Verification items for the finished model (mm, model axes). A direction names the side the tool comes from. Give positions to 0.01 mm unless a question says otherwise; leave off trailing zeros. Loops run counter-clockwise (first coordinate to the right, second up) from the corner with the lowest first, then second, coordinate; pieces in that order, holes last. Notation, with made-up numbers: (56, 37) - (63, 37) arc R21 ccw to (63, 41) - close; hole circle Ø11 at (-12, 60). An arc over 180 degrees is marked (long way). One line per item, written item: value. Start each with the question number.
1. Access from +Z, -Z, +X, -X, +Y, -Y to the whole of each face (thin tool, end or side, straight path). Record for faces 1 (the cylindrical face through (4.36, 2.45, 3.61)), 2 (the cylindrical face through (-0.1, -5, 3.6)), 3 (the flat face through (-0.1, -5.2, 3.2)), 4 (the cylindrical face through (-0.534, 4.065, 0.109)).
2. Scan lines: L1, parallel to Y at x = 0, z = 0.3; L2, parallel to Z at x = 2.5, y = -2; L3, parallel to X at y = -2.25, z = 0.35. Record each from-to range of solid material in increasing order. Write a range as [from, to].
3. Gauge pin test, flat ends, axial feed: pin 1 (1 mm diameter, centred on x = 1, z = 0, fed in from -Y); pin 2 (2 mm diameter, centred on y = 2, z = 0, fed in from -X); pin 3 (4.5 mm diameter, centred on x = 0, y = 6, fed in from -Z); pin 4 (2 mm diameter, centred on x = 0, y = 0, fed in from +Z). Record the tip position at first contact, or that the pin passes through.
4. Sectioned sample at A-A (x = 0). Count the separate pieces of the cut face and the enclosed holes in it, plus the area to 3 significant figures.
5. Mould release check, pull along X, two halves, no side actions. Record for faces 5 (the cylindrical face through (-4.3, 2.55, 3.61)), 6 (the flat face through (1, -1, 4)), 7 (the flat face through (-1, -1, 1.25)): pulls with the +X half, pulls with the -X half, needs draft (parallel to the pull), parting line crosses it, or undercut.
6. Sectioned sample at C-C (z = 2). Record the cut outline in (x, y).
from build123d import *

# Parameters (mm, degrees)
CYLINDER001_R     = 1.35
CYLINDER001_DEPTH = 10
ARRAY001_COUNT    = 3
CYLINDER_R        = 4.1
CYLINDER_DEPTH    = 2.25
SKETCH002_W       = 5
SKETCH002_H       = 4.7
ARRAY_Z_COUNT     = 6
ARRAY_Z_PITCH     = 1.6


with BuildPart() as obj1:
    # Cylinder001 → Cylinder001 (new body)
    with BuildSketch(Plane(origin=(0, 6, -4), x_dir=(1, 0, 0), z_dir=(0, 0, 1))):
        Circle(CYLINDER001_R)
    extrude(amount=CYLINDER001_DEPTH)

    # Array001: obj1 ×3 about axis
    array001_axis = Axis((0, 0, 0), (0, 0, 1))


with BuildPart() as obj1_1:
    add(obj1.part)
    for i in range(1, ARRAY001_COUNT):
        add(obj1.part.rotate(array001_axis, i * 360 / ARRAY001_COUNT))


with BuildPart() as lensfit:
    # Cylinder → Cylinder (new body)
    with BuildSketch(Plane.XY.offset(-1)):
        Circle(CYLINDER_R)
    extrude(amount=CYLINDER_DEPTH)


with BuildPart() as obj2:
    # Sketch002 → Revolution002 (revolve)
    with BuildSketch(Plane.XZ):
        with Locations((7.5, 0.85)):
            Rectangle(SKETCH002_W, SKETCH002_H)
    revolve(axis=Axis((0, 0, 0), (0, 0, 1)))


with BuildPart() as innergroovetool:
    # Sketch001 → Revolution001 (revolve)
    with BuildSketch(Plane.XZ):
        Polygon((4, 3.2), (4, 1.6), (8, 1.6), (8.8, 2.4), (8, 3.2), align=None)
    revolve(axis=Axis((0, 0, 0), (0, 0, 1)))

    # Array Z: InnerGrooveTool ×6


with BuildPart() as innergroovetool_1:
    add(innergroovetool.part)
    with Locations(*[(0, 0, -i * ARRAY_Z_PITCH) for i in range(1, ARRAY_Z_COUNT)]):
        add(innergroovetool.part)

    # Common: intersect obj2
    add(obj2.part, mode=Mode.INTERSECT)


with BuildPart() as boltcuts:
    # Sketch → Revolution (revolve)
    with BuildSketch(Plane.XZ):
        Polygon((1.25, 4), (1.25, -1.5), (8, -1.5), (8, 3.2), (5, 3.2), (5, 4), align=None)
    revolve(axis=Axis((0, 0, 0), (0, 0, 1)))

    # Fusion001: union InnerGrooveTool
    add(innergroovetool_1.part)

    # Cut: cut LensFit
    add(lensfit.part, mode=Mode.SUBTRACT)

    # Cut001: cut obj1
    add(obj1_1.part, mode=Mode.SUBTRACT)


solid = boltcuts.part
Results are:
1. face 1: +Z, +X
1. face 2: +Z, -Y
1. face 3: +Z
1. face 4: none
2. L1: y = [-8.3, -4.1], [4.1, 4.65], [7.35, 8.3]
2. L2: z = [-1.5, -1], [1.25, 4]
2. L3: x = [-8.04, -6.32], [-4.07, -3.43], [3.43, 4.07], [6.32, 8.04]
3. pin 1: stops at y = -8.44
3. pin 2: stops at x = -8.69
3. pin 3: stops at z = -1.5
3. pin 4: passes through
4. separate pieces: 3
4. enclosed holes: 0
4. area: 47.5 mm^2
5. face 5: pulls with the -X half
5. face 6: needs draft
5. face 7: undercut
6. outline: circle Ø16.8 at (0, 0); hole circle Ø2.7 at (-5.2, -3); hole circle Ø2.7 at (0, 6); hole circle Ø2.5 at (0, 0); hole circle Ø2.7 at (5.2, -3)
